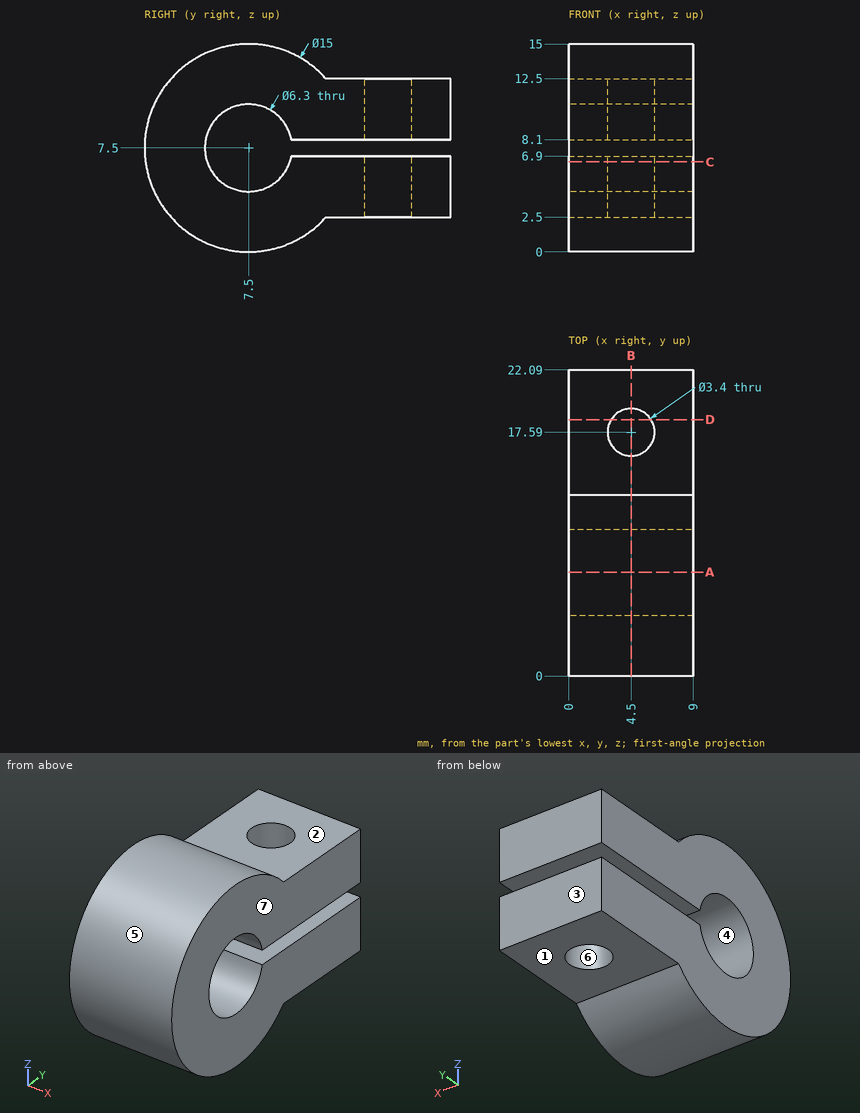
The figure shows three views and two pictorial views of one solid part (mm, origin at its lowest corner). Answer the questions. A direction names the side the tool comes from. Coordinates: 2 decimals unless noted, no trailing zeros. Loops run counter-clockwise (first coordinate to the right, second up) from the corner with the lowest first, then second, coordinate; pieces in that order, holes last. Notation, with made-up numbers: M 75.25,-2.5 L 107.25,-2.5 A17 cw 107.25,11.5 Z; hole C -26.75,-23.5 d11. An arc over 180 degrees is marked long. Use CSV: the item, a comma, the result in double quotes. Start each with the question number.
(1) For the marked faces 1, 2 and 3, determine the directions among +Z, -Z, +X, -X, +Y, -Y from which every point of the face is accessible in a straight line to the end or side of a thin tool.
(2) Find section B-B, the plane x = 4.5. Give the vertices of the cut face in (y, z).
(3) Find section D-D, the plane y = 18.5. Give the vertices of the cut face in (x, z).
(4) Consider line 1 (Z direction, x = 1, y = 20); line 2 (Y direction, x = 5.75, z = 10.25) (1 decimal); line 3 (Z direction, x = 5.75, y = 7.5). Determine where each line is inside the solid, lowest interval first.
(5) Given pin 1 Ø3 at (x, y) = (4.5, 17.59) entering from -Z; pin 2 Ø1 at (x, z) = (7.5, 13) entering from -Y; pin 3 Ø4.5 at (x, y) = (4, 17.5) entering from -Z; pin 4 Ø2 at (x, y) = (3, 3.5) entering from -Z, each flat-ended and moving along its own axis, determine where each tip first touches the part or whether it passes through.
(6) Find section C-C, the plane z = 6.5. Give the vertices of the cut face in (x, y).
(7) For a pull along Y with two mould halves and no side action, classify the marked faces 4, 5, 6 and 7 as +Y half, -Y half, draft (parallel to the pull), parting line (faces both ways), or undercut.
(8) Find section A-A, the plane y = 7.5. Give the vertices of the cut face in (x, z).
Recorded:
1,face 1,"-Z, +X, -X, +Y"
1,face 2,"+Z, +X, -X, +Y"
1,face 3,"+Z, -Z, +X, -X, +Y"
2,outline,"M 10.59,6.9 A3.15 cw long 10.59,8.1 L 15.89,8.1 L 15.89,12.5 L 13.09,12.5 A7.5 ccw long 13.09,2.5 L 15.89,2.5 L 15.89,6.9 Z; M 19.29,2.5 L 22.09,2.5 L 22.09,6.9 L 19.29,6.9 Z; M 19.29,8.1 L 22.09,8.1 L 22.09,12.5 L 19.29,12.5 Z"
3,outline,"M 0,2.5 L 3.06,2.5 L 3.06,6.9 L 0,6.9 Z; M 0,8.1 L 3.06,8.1 L 3.06,12.5 L 0,12.5 Z; M 5.94,2.5 L 9,2.5 L 9,6.9 L 5.94,6.9 Z; M 5.94,8.1 L 9,8.1 L 9,12.5 L 5.94,12.5 Z"
4,line 1,"z = 2.5 to 6.9, 8.1 to 12.5"
4,line 2,"y = 0.5 to 6, 9 to 16.4, 18.7 to 22.1"
4,line 3,"z = 0 to 4.35, 10.65 to 15"
5,pin 1,"passes through"
5,pin 2,"stops at y = 1.91"
5,pin 3,"stops at z = 2.5"
5,pin 4,"stops at z = 0.63"
6,outline,"M 0,0.07 L 9,0.07 L 9,4.51 L 0,4.51 Z; M 0,10.49 L 9,10.49 L 9,22.09 L 0,22.09 Z; hole C 4.5,17.59 d3.4"
7,face 4,"undercut"
7,face 5,"parting line"
7,face 6,"undercut"
7,face 7,"draft"
8,outline,"M 0,0 L 9,0 L 9,4.35 L 0,4.35 Z; M 0,10.65 L 9,10.65 L 9,15 L 0,15 Z"
